Answer from the drawing. Dimensions are ordinates in mm from the lowest x, y and z of the part. Give positions to 0.01 mm unless a question says otherwise; leave off trailing zeros. Order: outer loops, then holes, each group sorted by start corner. A loop starts at its lowest first (then second) coordinate and runs counter-clockwise, first axis right, second up. Notation, with made-up numbers: (49, 17.5) -> (80, 17.5) arc R16 cw to (80, 43.5) -> close; hole circle Ø3 at (40.25, -32.5). An arc over 180 degrees is marked (long way). Answer as a JSON object with one key per item and string values. Group by question number.
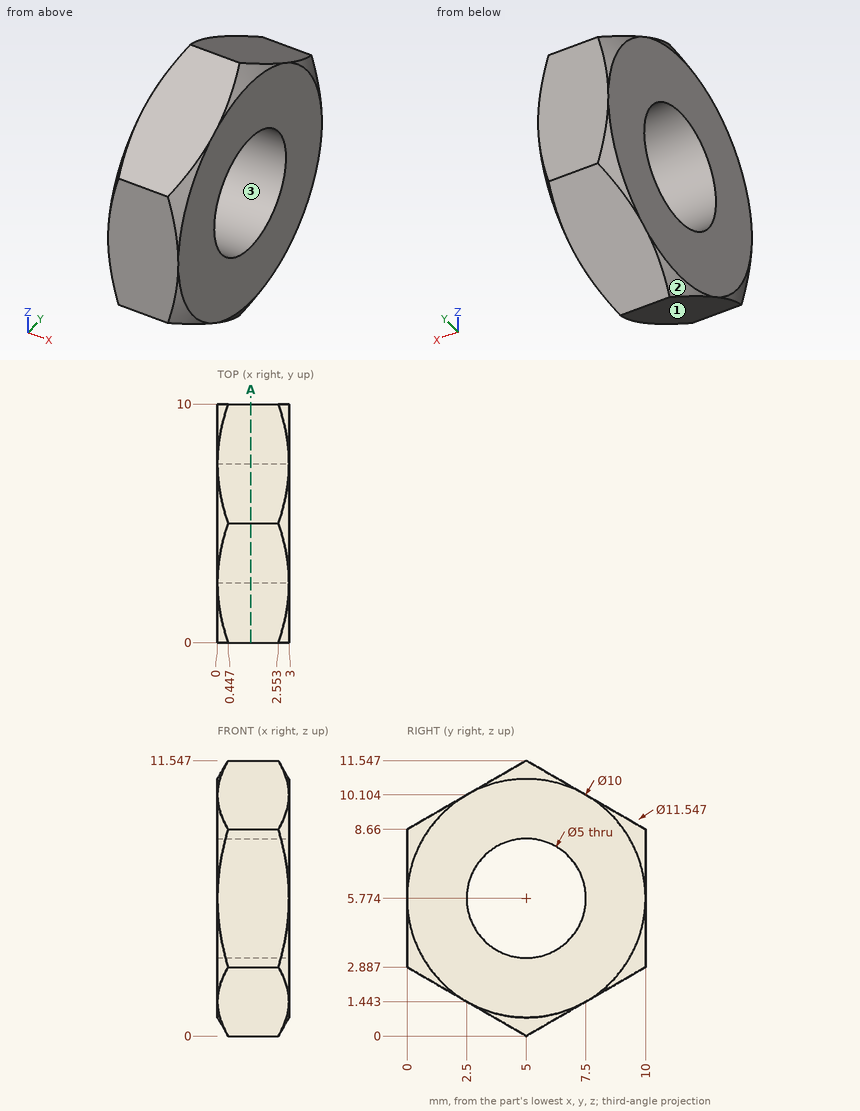
(1) For a pull along Y with two mould halves and no side action, classify the marked faces 1, 2 and 3 as +Y half, -Y half, draft (parallel to the pull), parting line (faces both ways), or undercut.
(2) A cutting plane is placed at A-A (x = 1.4). Determine the outline of the cut face in (y, z).
(3) Find the intervals of material crossed by line 1 along Y through (x, z) = (0.8, 5.75); line 2 along Y through (x, z) = (0.2, 7.25) (1 decimal); line 3 along Y through (x, z) = (0.35, 1.5) (1 decimal), in increasing order. Write a range as [from, to].
Check sheet entries:
{
 "1": {"face 1": "-Y half", "face 2": "parting line", "face 3": "undercut"},
 "2": {"outline": "(0, 2.89) -> (5, 0) -> (10, 2.89) -> (10, 8.66) -> (5, 11.55) -> (0, 8.66) -> close; hole circle Ø5 at (5, 5.77)"},
 "3": {"line 1": "y = [0, 2.5], [7.5, 10]", "line 2": "y = [0, 3], [7, 10]", "line 3": "y = [2.4, 7.6]"}
}
